Check sheet for the modelled part. Datum: model origin and axes. Units: mm. Face numbers are marked on the shaded views. A direction names the side the tool comes from. Round coordinates to 2 decimals unless told otherwise and drop trailing zeros. Loops run counter-clockwise (first coordinate to the right, second up) from the corner with the lowest first, then second, coordinate; pieces in that order, holes last. Notation, with made-up numbers: (42.5, 6.5) -> (71.5, 6.5) arc R18 ccw to (71.5, 37.5) -> close; hole circle Ø1 at (41.25, 13.25). An arc over 180 degrees is marked (long way). Use one line per item in the form item = value. Start each with the question number.
(1) Sectioned sample at C-C (x = 0.5). Record the cut outline in (y, z).
(2) Go/stop test with flat-tipped pins: pin 1 (2 mm diameter, centred on x = 3, y = -2.5, fed in from -Z); pin 2 (10 mm diameter, centred on y = 5, z = 14, fed in from +X); pin 3 (2 mm diameter, centred on x = 2, z = 6.5, fed in from +Y). Record where each tip stops, or that it passes through.
(3) Draft check along Z on the marked faces 3, 4 and 5. Enter one of: released by +Z, released by -Z, zero draft, split by the parting line, or undercut.
(4) Set-up check for the marked faces 1 and 2: record each of +Z, -Z, +X, -X, +Y, -Y from which the full face is reachable in a straight line by a thin tool's end or side.
(5) Sectioned sample at B-B (x = 5.5). Record the cut outline in (y, z), and give its area (3 significant figures).
(6) Material ranges on probe 1 along Z at (x, y) = (5, 0); probe 2 along Z at (x, y) = (6.75, -4.5); probe 3 along Y at (x, z) = (2.5, 2), recorded low to high. Write a range as [from, to].
(7) Sectioned sample at A-A (y = 0). State how many separate pieces and enclosed holes the cut face has, and give its area (3 significant figures).
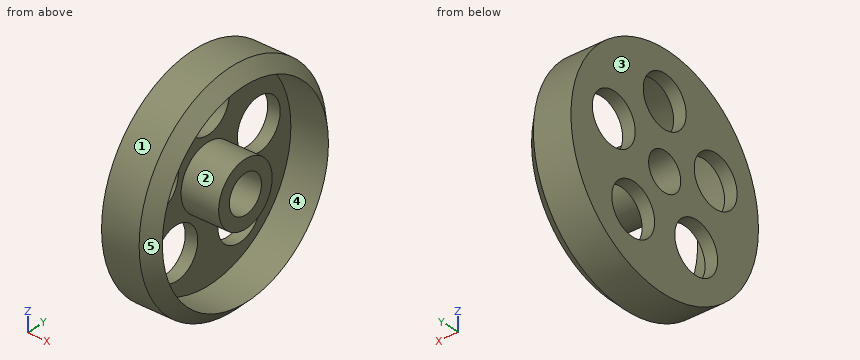
from build123d import *

# Parameters (mm, degrees)
F0_W            = 8
F0_H            = 17.5
F3_D            = 6
F3_DEPTH        = 12
F3_TIP          = 1.8025818571
F4_T            = -2
F6_D            = 8
F6_DEPTH        = 12
F6_TIP          = 2.4034424761
F6_COPIES_COUNT = 5
F7_SIZE         = 1.99999


# Not quite as in the source:
# - a fillet or chamfer is up to 0.001 mm smaller than in the source, because OpenCascade refuses the exact size
# - a pattern or mirror of a feature is missing from the dataset's text; its kind, count and spacing are read off the source's solid


with BuildPart() as f1:
    # F0 (on Top) → F1 (revolve)
    with BuildSketch(Plane.XY):
        with Locations((4, 8.75)):
            Rectangle(F0_W, F0_H)
    revolve(axis=Axis((4, 0, 0), (1, 0, 0)))

    # F3
    with Locations(Plane(origin=(0, 0, 0), x_dir=(0, 1, 0), z_dir=(-1, 0, 0))):
        with Locations((0, 0)):
            Hole(F3_D / 2, depth=F3_DEPTH)
            with Locations((0, 0, -(F3_DEPTH + F3_TIP / 2))):  # 118° drill point
                Cone(0, F3_D / 2, F3_TIP, mode=Mode.SUBTRACT)

    # F4
    f4_openings = [f1.faces().sort_by_distance(p)[0] for p in [
        (8, -17.005025, 0),
    ]]
    offset(amount=F4_T, openings=f4_openings)

    # F6
    with Locations(Plane(origin=(0, 0, 0), x_dir=(0, 1, 0), z_dir=(-1, 0, 0))):
        with Locations((0, -10)):
            f6 = Hole(F6_D / 2, depth=F6_DEPTH)
            with Locations((0, 0, -(F6_DEPTH + F6_TIP / 2))):  # 118° drill point
                Cone(0, F6_D / 2, F6_TIP, mode=Mode.SUBTRACT)

    # F6_copies: F6 ×5 about axis
    f6_copies_axis = Axis((0, 0, 0), (1, 0, 0))
    for i in range(1, F6_COPIES_COUNT):
        add(f6.rotate(f6_copies_axis, i * 360 / F6_COPIES_COUNT), mode=Mode.SUBTRACT)

    # F7 (size 2 in the source; OpenCascade refuses exactly that, so slightly less here)
    f7_edges = [f1.edges().sort_by_distance(p)[0] for p in [
        (8, -17.5, 0),
    ]]
    chamfer(f7_edges, length=F7_SIZE)


solid = f1.part
Checks:
q1.outline = circle Ø35 at (0, 0); hole circle Ø8 at (-9.51, 3.09); hole circle Ø8 at (-5.88, -8.09); hole circle Ø8 at (0, 10); hole circle Ø6 at (0, 0); hole circle Ø8 at (5.88, -8.09); hole circle Ø8 at (9.51, 3.09)
q2.pin_1 = -17.44
q2.pin_2 = 8
q2.pin_3 = 16.61
q3.face_3 = zero draft
q3.face_4 = undercut
q3.face_5 = split by the parting line
q4.face_1 = +X, -X
q4.face_2 = +X
q5.outline = circle Ø35 at (0, 0); circle Ø10 at (0, 0); hole circle Ø31 at (0, 0); hole circle Ø6 at (0, 0)
q5.area = 258 mm2
q6.probe_1 = [-17.5, -15.5], [-5, -3], [3, 5], [15.5, 17.5]
q6.probe_2 = [-16.13, -14.83], [-2.18, 2.18], [14.83, 16.13]
q6.probe_3 = [-17.39, -15.37], [-4.58, -2.24], [2.24, 4.58], [15.37, 17.39]
q7.separate_pieces = 3
q7.enclosed_holes = 0
q7.area = 86.0 mm2
